from build123d import *

# Parameters (mm, degrees)
BOSS_EXTRUDE1_DEPTH = 5.5
SKETCH2_W           = 3
SKETCH2_H           = 1.5
SKETCH2_W_2         = 1.358942276
SKETCH2_H_2         = 1.316057296
CUT_EXTRUDE1_DEPTH  = 1
SKETCH3_W           = 0.2
SKETCH3_H           = 0.57
BOSS_EXTRUDE2_DEPTH = 3.75
SKETCH4_W           = 1.421686747
SKETCH4_H           = 0.409638554
CUT_EXTRUDE2_DEPTH  = 0.1


with BuildPart() as part:
    # Sketch1 → Boss-Extrude1 (new body)
    with BuildSketch(Plane.XY):
        Polygon((-4.985, -2.01), (-1.5, -2.01), (-1.5, -1.71), (1.5, -1.71), (1.5, -2.01), (4.985, -2.01), (4.985, 2.01), (-4.985, 2.01), align=None)
    extrude(amount=BOSS_EXTRUDE1_DEPTH)

    # Sketch2 → Cut-Extrude1 (cut)
    with BuildSketch(Plane.XY.offset(5.5)):
        Rectangle(SKETCH2_W, SKETCH2_H)
        with Locations((0.741156602, 0)):
            Rectangle(SKETCH2_W_2, SKETCH2_H_2, mode=Mode.SUBTRACT)
    extrude(amount=-CUT_EXTRUDE1_DEPTH, mode=Mode.SUBTRACT)

    # Sketch3 → Boss-Extrude2 (add)
    with BuildSketch(Plane(origin=(0, 0, 0), x_dir=(-1, 0, 0), z_dir=(0, 0, -1))):
        with Locations((-4, 0)):
            Rectangle(SKETCH3_W, SKETCH3_H)
        with Locations((4, 0)):
            Rectangle(SKETCH3_W, SKETCH3_H)
    extrude(amount=BOSS_EXTRUDE2_DEPTH)

    # Sketch4 → Cut-Extrude2 (cut)
    # profile 1 of 3: a face of its own
    with BuildSketch(Plane.XY.offset(5.5)):
        with BuildLine():
            Line((-2.353314341, 1.216281942), (-2.353314341, 0.956492785))
            Line((-2.353314341, 0.956492785), (-3.611973979, 0.498284954))
            add(Edge.make_bspline(
                [(-3.611973979, 0.498284954), (-3.597433311, 0.501148384), (-3.570177198, 0.50651581), (-3.531507992, 0.512558558), (-3.497858896, 0.516745674), (-3.476943559, 0.517254487), (-3.467395666, 0.517486761)],
                knots=[0, 0, 0, 0, 1.217419203, 2.282021413, 3.215739318, 4, 4, 4, 4], degree=3))
            Line((-3.467395666, 0.517486761), (-2.353314341, 0.517486761))
            Line((-2.353314341, 0.517486761), (-2.353314341, 0.228330135))
            Line((-2.353314341, 0.228330135), (-4.353314341, 0.228330135))
            Line((-4.353314341, 0.228330135), (-4.353314341, 0.488119291))
            Line((-4.353314341, 0.488119291), (-3.120257112, 0.946327123))
            add(Edge.make_bspline(
                [(-3.120257112, 0.946327123), (-3.134669922, 0.943449375), (-3.161913736, 0.938009714), (-3.200482023, 0.932125999), (-3.234118261, 0.927844891), (-3.254910338, 0.927351775), (-3.264458919, 0.927125315)],
                knots=[0, 0, 0, 0, 1.210373155, 2.287907843, 3.213736571, 4, 4, 4, 4], degree=3))
            Line((-3.264458919, 0.927125315), (-4.353314341, 0.927125315))
            Line((-4.353314341, 0.927125315), (-4.353314341, 1.216281942))
            Line((-4.353314341, 1.216281942), (-2.353314341, 1.216281942))
        make_face()
    # profile 2 of 3: a face of its own
    with BuildSketch(Plane.XY.offset(5.5)):
        with BuildLine():
            add(Edge.make_bspline(
                [(-2.511070365, -0.036730106), (-2.49908555, -0.037580702), (-2.476448953, -0.039187284), (-2.444890766, -0.047711625), (-2.417445544, -0.060219475), (-2.395243748, -0.078659514), (-2.376803709, -0.10086131), (-2.364295859, -0.128306532), (-2.355771519, -0.159864718), (-2.354164936, -0.182501315), (-2.353314341, -0.19448613)],
                knots=[0, 0, 0, 0, 1.144701434, 2.162081395, 3.105417678, 4, 4.894582322, 5.837918605, 6.855298566, 8, 8, 8, 8], degree=3))
            Line((-2.353314341, -0.19448613), (-2.353314341, -0.866925889))
            add(Edge.make_bspline(
                [(-2.353314341, -0.866925889), (-2.354164936, -0.878910704), (-2.355771519, -0.901547302), (-2.364295859, -0.933105488), (-2.376803709, -0.96055071), (-2.395243748, -0.982752506), (-2.417445544, -1.001192545), (-2.444890766, -1.013700395), (-2.476448953, -1.022224736), (-2.49908555, -1.023831318), (-2.511070365, -1.024681914)],
                knots=[0, 0, 0, 0, 1.144701434, 2.162081395, 3.105417678, 4, 4.894582322, 5.837918605, 6.855298566, 8, 8, 8, 8], degree=3))
            Line((-2.511070365, -1.024681914), (-4.195558317, -1.024681914))
            add(Edge.make_bspline(
                [(-4.195558317, -1.024681914), (-4.207543132, -1.023831318), (-4.230179729, -1.022224736), (-4.261737915, -1.013700395), (-4.289183137, -1.001192545), (-4.311384933, -0.982752506), (-4.329824972, -0.96055071), (-4.342332823, -0.933105488), (-4.350857163, -0.901547302), (-4.352463745, -0.878910704), (-4.353314341, -0.866925889)],
                knots=[0, 0, 0, 0, 1.144701434, 2.162081395, 3.105417678, 4, 4.894582322, 5.837918605, 6.855298566, 8, 8, 8, 8], degree=3))
            Line((-4.353314341, -0.866925889), (-4.353314341, -0.19448613))
            add(Edge.make_bspline(
                [(-4.353314341, -0.19448613), (-4.352463745, -0.182501315), (-4.350857163, -0.159864718), (-4.342332823, -0.128306532), (-4.329824972, -0.10086131), (-4.311384933, -0.078659514), (-4.289183137, -0.060219475), (-4.261737915, -0.047711625), (-4.230179729, -0.039187284), (-4.207543132, -0.037580702), (-4.195558317, -0.036730106)],
                knots=[0, 0, 0, 0, 1.144701434, 2.162081395, 3.105417678, 4, 4.894582322, 5.837918605, 6.855298566, 8, 8, 8, 8], degree=3))
            Line((-4.195558317, -0.036730106), (-2.511070365, -0.036730106))
        make_face()
        with Locations((-3.35331434, -0.53070601)):
            Rectangle(SKETCH4_W, SKETCH4_H, mode=Mode.SUBTRACT)
    # profile 3 of 3: a face of its own
    with BuildSketch(Plane.XY.offset(5.5)):
        Polygon((4.152608675, 0.176962569), (4.152608675, -0.112194057), (2.730921928, -0.112194057), (2.730921928, -0.232675985), (2.694777349, -0.232675985), (2.152608675, -0.072660924), (2.152608675, 0.176962569), align=None)
    extrude(amount=-CUT_EXTRUDE2_DEPTH, mode=Mode.SUBTRACT)


solid = part.part
Model file for the job. Use its own axes, mm. A direction names the side the tool comes from. Coordinates: 2 decimals unless noted, no trailing zeros. Order: outer loops, then holes, each group sorted by start corner. A loop starts at its lowest first (then second) coordinate and runs counter-clockwise, first axis right, second up. Notation, with made-up numbers: (84, 64) -> (97, 64) arc R11 ccw to (97, 70) -> close; hole circle Ø4 at (28.5, 31). An arc over 180 degrees is marked (long way). Return JSON: item names as keys, results as strings. Group by question number.
Item 1: Pull direction Y, two halves, no side cores. Call faces 1 (the flat face through (0.062, 0, 5)), 2 (the flat face through (0, 2.01, 3)), 3 (the flat face through (0, -1.71, 3)), 4 (the flat face through (-4.985, 0, 3)): pulls with the +Y half, pulls with the -Y half, needs draft (parallel to the pull), parting line crosses it, or undercut.
Item 2: Tool access for faces 5 (the flat face through (1, 0, 5.5)), 6 (the flat face through (-1.5, 0, 5)): list every direction of +Z, -Z, +X, -X, +Y, -Y with a clear straight run to the whole face (end or side of a thin tool).
Item 3: Saw through at D-D on x = -3.75. Write the cut outline in (y, z), then the cut area to 3 significant figures.
Item 4: Saw through at A-A on z = -2.75. Write the cut outline in (x, y) (3 decimals).
Item 5: Saw through at B-B on y = 1.1. Write the cut outline in (x, z) (3 decimals), then the cut area to 3 significant figures.
Item 6: Flat gauge pin, fed straight in: P1, Ø1.5, axis at x = 2, y = -0.5, coming from the -Z side. Where does the tip first touch, or does it go through?
Item 7: Saw through at C-C on z = 1. Write the cut outline in (x, y) (3 decimals).
Item 8: Wall check: line 1 along Z through (x, y) = (-2.5, 1.35); line 2 along Z through (x, y) = (-4, -0.9); line 3 along Y through (x, z) = (1.25, 3). Give the ranges that are in metal, low to high. Write a range as [from, to].
Values found:
{
 "1": {"face 1": "undercut", "face 2": "pulls with the +Y half", "face 3": "pulls with the -Y half", "face 4": "needs draft"},
 "2": {"face 5": "+Z, +X, -X, +Y, -Y", "face 6": "+Z"},
 "3": {"outline": "(-2.01, 0) -> (2.01, 0) -> (2.01, 5.5) -> (1.22, 5.5) -> (1.22, 5.4) -> (0.93, 5.4) -> (0.93, 5.5) -> (0.71, 5.5) -> (0.71, 5.4) -> (0.23, 5.4) -> (0.23, 5.5) -> (-0.04, 5.5) -> (-0.04, 5.4) -> (-0.33, 5.4) -> (-0.33, 5.5) -> (-0.74, 5.5) -> (-0.74, 5.4) -> (-1.02, 5.4) -> (-1.02, 5.5) -> (-2.01, 5.5) -> close", "area": "22.0 mm2"},
 "4": {"outline": "(-4.1, -0.285) -> (-3.9, -0.285) -> (-3.9, 0.285) -> (-4.1, 0.285) -> close; (3.9, -0.285) -> (4.1, -0.285) -> (4.1, 0.285) -> (3.9, 0.285) -> close"},
 "5": {"outline": "(-4.985, 0) -> (4.985, 0) -> (4.985, 5.5) -> (-2.353, 5.5) -> (-2.353, 5.4) -> (-4.353, 5.4) -> (-4.353, 5.5) -> (-4.985, 5.5) -> close", "area": "54.6 mm2"},
 "6": {"P1": "stops at z = 0"},
 "7": {"outline": "(-4.985, -2.01) -> (-1.5, -2.01) -> (-1.5, -1.71) -> (1.5, -1.71) -> (1.5, -2.01) -> (4.985, -2.01) -> (4.985, 2.01) -> (-4.985, 2.01) -> close"},
 "8": {"line 1": "z = [0, 5.5]", "line 2": "z = [0, 5.4]", "line 3": "y = [-1.71, 2.01]"}
}
